```python
from build123d import *

# Parameters (mm, degrees)
SKETCH1_W           = 1920
SKETCH1_H           = 1994
BOSS_EXTRUDE1_DEPTH = 120
SKETCH2_W           = 60
SKETCH2_H           = 60
CUT_EXTRUDE1_DEPTH  = 2167.750793239


with BuildPart() as part:
    # Sketch1 → Boss-Extrude1 (new body)
    with BuildSketch(Plane(origin=(0, 0, 0), x_dir=(1, 0, 0), z_dir=(0, 1, 0))):
        Rectangle(SKETCH1_W, SKETCH1_H)
    extrude(amount=BOSS_EXTRUDE1_DEPTH)

    # Sketch2 → Cut-Extrude1 (cut, through all)
    with BuildSketch(Plane.ZY.offset(960)):
        with Locations((-967, 90)):
            Rectangle(SKETCH2_W, SKETCH2_H)
        with Locations((967, 90)):
            Rectangle(SKETCH2_W, SKETCH2_H)
    extrude(amount=-CUT_EXTRUDE1_DEPTH, mode=Mode.SUBTRACT)


solid = part.part
```
Could you check a few things on this model? Use its own coordinates, in mm. A direction names the side the tool comes from. Round coordinates to 2 decimals unless told otherwise and drop trailing zeros. Loops run counter-clockwise (first coordinate to the right, second up) from the corner with the lowest first, then second, coordinate; pieces in that order, holes last. Notation, with made-up numbers: (11, 12) - (59, 12) arc R5 ccw to (59, 18) - close; hole circle Ø9 at (88.5, 1.25). An arc over 180 degrees is marked (long way). Answer in a Markdown table with one row per item. Add a question column.
(1) I'm going to push flat-ended pins straight in: pin 1 (3 mm diameter, centred on x = 348, y = 89, fed in from -Z); pin 2 (18 mm diameter, centred on x = -221, z = -959.5, fed in from +Y). Where does each tip first touch, or does it pass through?
(2) I need wall thicknesses on line 1 along Z through (x, y) = (-573, 102.5). Which ranges of the line are inside material? Lowest first, please.
(3) For faces 1 (the face through (-13, 120, -13)), 2 (the face through (-13, 90, -937)), 3 (the face through (-13, 60, 967)), which set-ups out of +Z, -Z, +X, -X, +Y, -Y let a thin tool reach every point of the face, with its end or its side?
(4) If we section it at B-B (y = 81): Please give me the cut outline in (x, z).
(5) If we section it at A-A (x = -105): Please give me the cut outline in (y, z), plus the area to 3 significant figures.
Model answer:
| question | item | result |
|---|---|---|
| 1 | pin 1 | stops at z = -937 |
| 1 | pin 2 | stops at y = 60 |
| 2 | line 1 | z = -937 to 937 |
| 3 | face 1 | +Z, -Z, +X, -X, +Y |
| 3 | face 2 | -Z, +X, -X, +Y |
| 3 | face 3 | +Z, +X, -X, +Y |
| 4 | outline | (-960, -937) - (960, -937) - (960, 937) - (-960, 937) - close |
| 5 | outline | (0, -997) - (60, -997) - (60, -937) - (120, -937) - (120, 937) - (60, 937) - (60, 997) - (0, 997) - close |
| 5 | area | 232,000 mm² |
